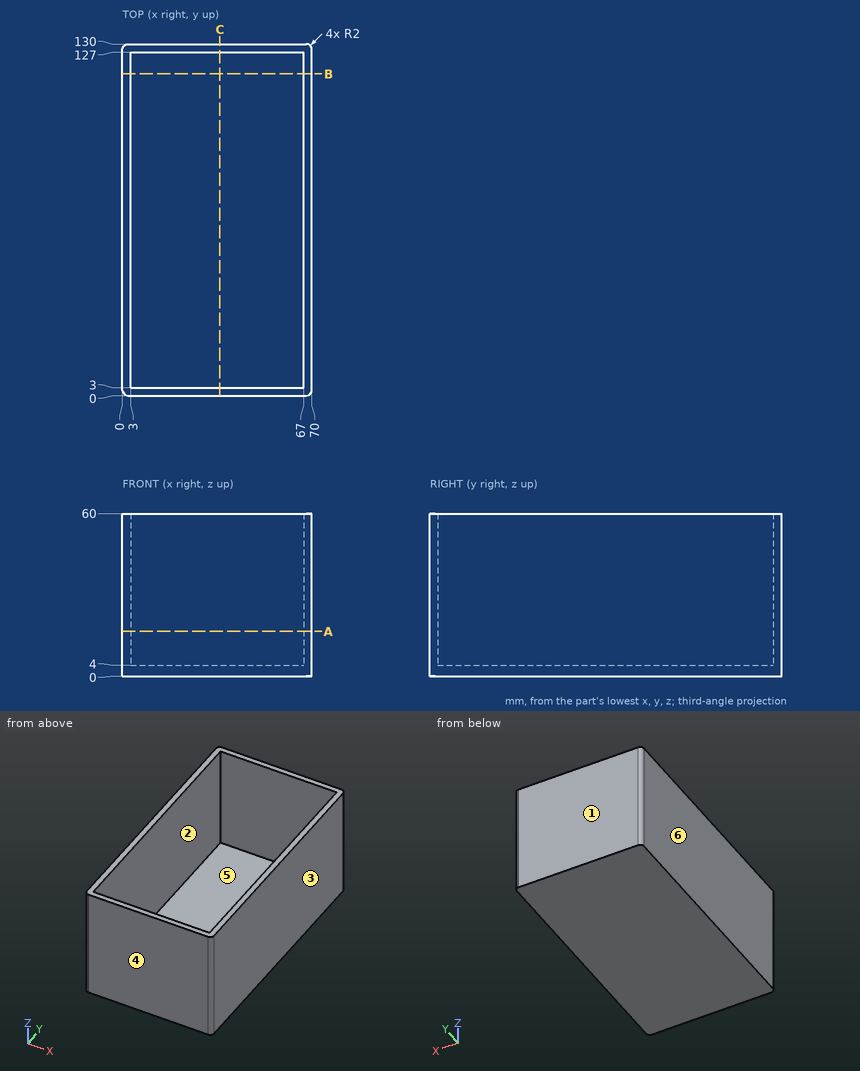
Geometry: see drawing. Coordinates: mm, zero at the bounding-box minimum. A direction names the side the tool comes from. Give positions to 0.01 mm unless a question says otherwise; leave off trailing zeros. Loops run counter-clockwise (first coordinate to the right, second up) from the corner with the lowest first, then second, coordinate; pieces in that order, holes last. Notation, with made-up numbers: M 2.25,41.5 L 40.25,41.5 A17 ccw 40.25,63.5 Z; hole C -0.5,-18.75 d7. An arc over 180 degrees is marked long. Use one line per item in the form item = value.
1. Reachability of the marked faces 5 and 6 from +Z, -Z, +X, -X, +Y, -Y: full face, straight path, thin tool, end or side. Return the list, or none.
Numbers:
face_5 = +Z
face_6 = +Z, -Z, -X, +Y, -Y
2. Section query A-A, the plane z = 16.5. Return the cut outline in (x, y), and give its area (3 significant figures).
Numbers:
outline = M 0,2 A2 ccw 2,0 L 68,0 A2 ccw 70,2 L 70,128 A2 ccw 68,130 L 2,130 A2 ccw 0,128 Z; hole M 3,3 L 67,3 L 67,127 L 3,127 Z
area = 1,160 mm²
3. First-contact query: pin 1 (6 mm diameter, centred on x = 26, y = 94.5, fed in from +Z). Flat tip, straight axial feed; report the tip coordinate or a pass-through.
Numbers:
pin_1 = 4
4. Line query: L1, parallel to X at y = 25, z = 16; L2, parallel to Y at x = 57.5, z = 7.5; L3, parallel to Z at x = 10.5, y = 58.5. Output: solid intervals per line, ascending.
Numbers:
L1 = 0 to 3, 67 to 70
L2 = 0 to 3, 127 to 130
L3 = 0 to 4
5. Section query C-C, the plane x = 36. Return the cut outline in (y, z).
Numbers:
outline = M 0,0 L 130,0 L 130,60 L 127,60 L 127,4 L 3,4 L 3,60 L 0,60 Z
6. Pull-direction query (Y, two-part tool) for the marked faces 1, 2, 3 and 4; classes: released by +Y, released by -Y, zero draft, split by the parting line, or undercut.
Numbers:
face_1 = released by +Y
face_2 = undercut
face_3 = zero draft
face_4 = released by -Y
7. Section query B-B, the plane y = 119. Return the cut outline in (x, z), and give its area (3 significant figures).
Numbers:
outline = M 0,0 L 70,0 L 70,60 L 67,60 L 67,4 L 3,4 L 3,60 L 0,60 Z
area = 616 mm²
